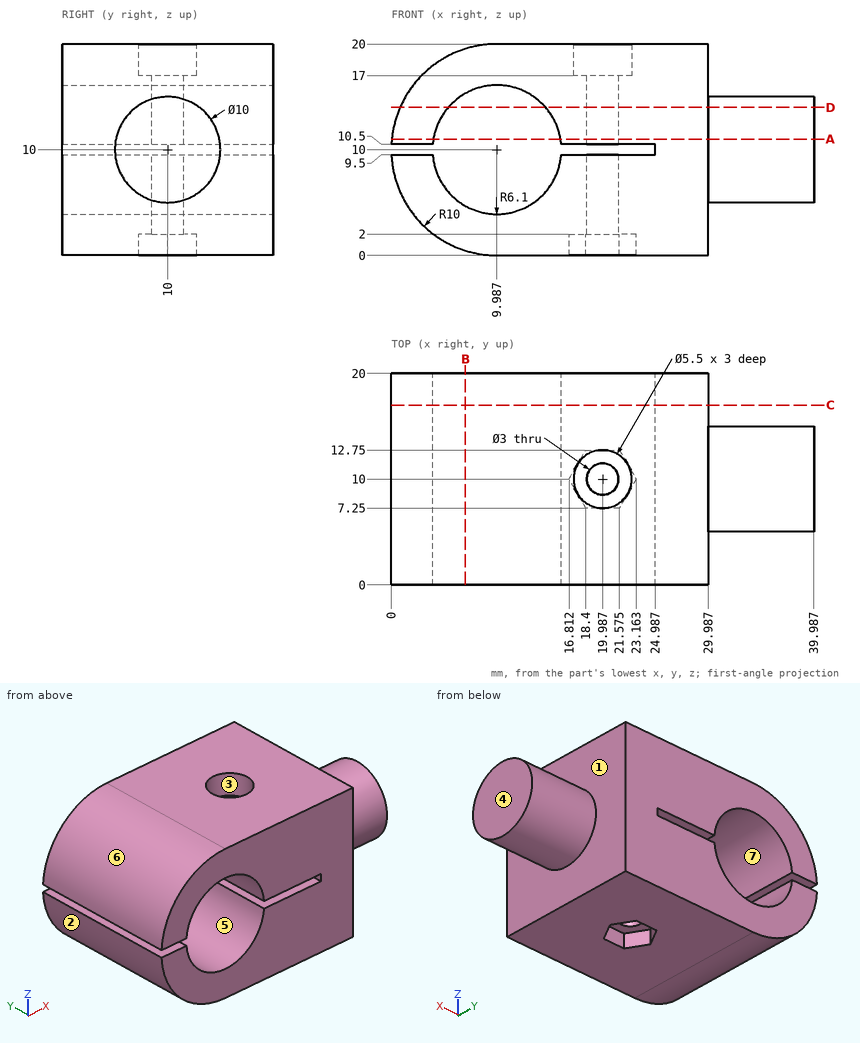
Part print with two shaded views. Sizes in mm from the minimum x, y, z corner. A direction names the side the tool comes from. Coordinates: 2 decimals unless noted, no trailing zeros. Order: outer loops, then holes, each group sorted by start corner. A loop starts at its lowest first (then second) coordinate and runs counter-clockwise, first axis right, second up. Notation, with made-up numbers: (-37, -6.75) - (-7, -6.75) arc R19 cw to (-7, 28.25) - close; hole circle Ø3 at (-38.5, 65). An arc over 180 degrees is marked (long way). Write item = value, one per line. Start each with the question number.
1) Saw through at D-D on z = 14. Write the cut outline in (x, y).
2) Two-plate mould, pull along Z, no slides. Class the marked faces 4, 5, 6 and 7: pulls with the +Z half, pulls with the -Z half, needs draft (parallel to the pull), parting line crosses it, or undercut.
3) Saw through at C-C on y = 17. Write the cut outline in (x, z).
4) Saw through at A-A on z = 11. Write the cut outline in (x, y) (1 decimal), then the cut area to 3 significant figures.
5) Wall check: line 1 along X through (y, z) = (9.75, 8.75) (1 decimal); line 2 along Z through (x, y) = (16.5, 16.5); line 3 along Z through (x, y) = (18.5, 7.75). Give the ranges that are in metal, low to high. Write a range as from..to.
6) Saw through at B-B on x = 7. Write the cut outline in (y, z), then the cut area to 3 significant figures.
7) Flat gauge pins, fed straight in: pin 1 Ø1 at (y, z) = (17, 18) entering from +X; pin 2 Ø2.5 at (x, y) = (19.99, 10) entering from -Z; pin 3 Ø1 at (x, y) = (35, 14) entering from -Z; pin 4 Ø1.2 at (x, y) = (1.5, 13) entering from +Z (1 decimal). Where does each tip first touch, or does it go through?
8) 3-axis set-ups, long thin cutter, end or side, ignore diameter. For the marked faces 1, 2 and 3: which of +Z, -Z, +X, -X, +Y, -Y reach the whole face in a straight line?
From the geometry:
q1.outline = (0.82, 0) - (5.38, 0) - (5.38, 20) - (0.82, 20) - close; (14.59, 0) - (29.99, 0) - (29.99, 7) - (39.99, 7) - (39.99, 13) - (29.99, 13) - (29.99, 20) - (14.59, 20) - close; hole circle Ø3 at (19.99, 10)
q2.face_4 = needs draft
q2.face_5 = undercut
q2.face_6 = pulls with the +Z half
q2.face_7 = undercut
q3.outline = (0, 9.5) arc R10 ccw to (9.99, 0) - (29.99, 0) - (29.99, 20) - (9.99, 20) arc R10 ccw to (0, 10.5) - (3.91, 10.5) arc R6.1 cw to (16.07, 10.5) - (24.99, 10.5) - (24.99, 9.5) - (16.07, 9.5) arc R6.1 cw to (3.91, 9.5) - close
q4.outline = (0, 0) - (4, 0) - (4, 20) - (0, 20) - close; (16, 0) - (30, 0) - (30, 5.1) - (40, 5.1) - (40, 14.9) - (30, 14.9) - (30, 20) - (16, 20) - close; hole circle Ø3 at (20, 10)
q4.area = 449 mm^2
q5.line_1 = 0.1..4, 16..18.5, 21.5..40
q5.line_2 = 0..9.5, 10.5..20
q5.line_3 = 2..9.5, 10.5..17
q6.outline = (0, 0.46) - (20, 0.46) - (20, 4.68) - (0, 4.68) - close; (0, 15.32) - (20, 15.32) - (20, 19.54) - (0, 19.54) - close
q6.area = 169 mm^2
q7.pin_1 = 29.99
q7.pin_2 = through
q7.pin_3 = 6.43
q7.pin_4 = 16.1
q8.face_1 = +X
q8.face_2 = -Z, -X, +Y, -Y
q8.face_3 = +Z
